For this review, use the dimensioned drawing (mm, ordinates from the lowest corner) and the shaded views. A direction names the side the tool comes from. Give positions to 0.01 mm unless a question says otherwise; leave off trailing zeros. Loops run counter-clockwise (first coordinate to the right, second up) from the corner with the lowest first, then second, coordinate; pieces in that order, holes last. Notation, with made-up numbers: (67.5, 84.25) - (94.5, 84.25) arc R19 ccw to (94.5, 115.25) - close; hole circle Ø3 at (-36, 7). An arc over 180 degrees is marked (long way). Put each result on its own line as item: value.
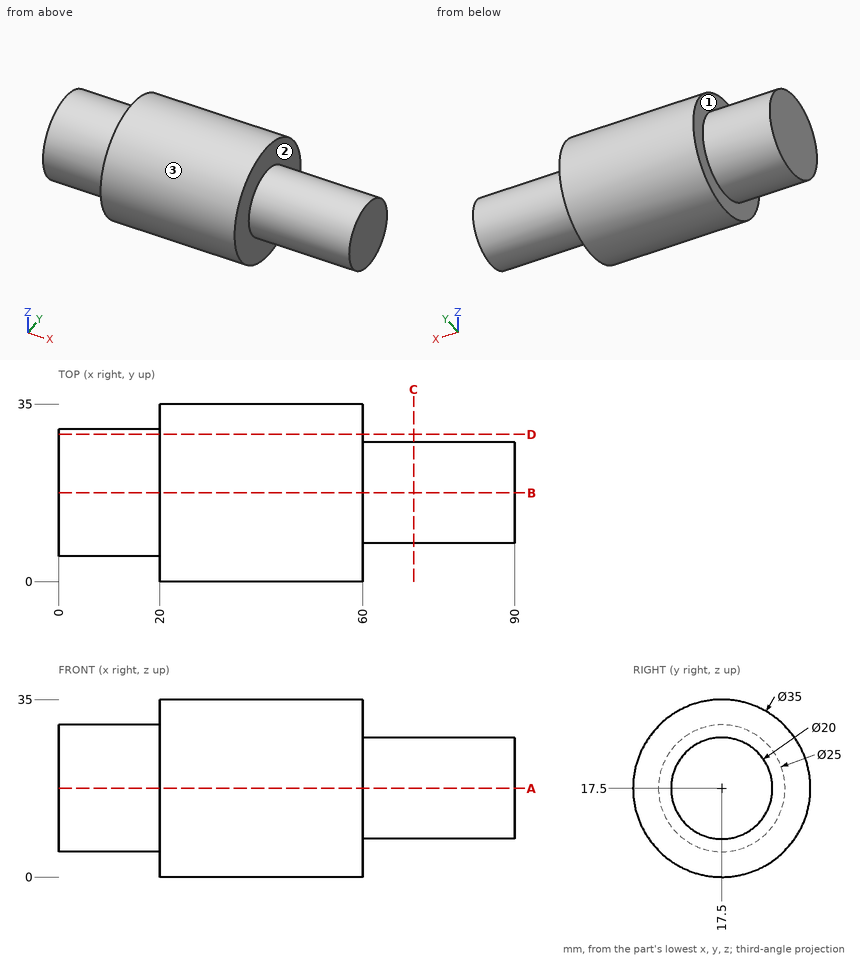
1) For the marked faces 1, 2 and 3, list the 3-axis set-ups (+Z, -Z, +X, -X, +Y, -Y) from which the entire face can be reached by the end or side of a thin tool; tool diameter is ignored.
Geometry check:
face 1: -X
face 2: +X
face 3: +X, -X
2) Take a section at A-A on z = 17.5. State the section outline as (x, y) points, and give its area (3 significant figures).
Geometry check:
outline: (0, 5) - (20, 5) - (20, 0) - (60, 0) - (60, 7.5) - (90, 7.5) - (90, 27.5) - (60, 27.5) - (60, 35) - (20, 35) - (20, 30) - (0, 30) - close
area: 2,500 mm²
3) Take a section at D-D on y = 29. State the section outline as (x, z) points, and give its area (3 significant figures).
Geometry check:
outline: (0, 12.6) - (20, 12.6) - (20, 4.31) - (60, 4.31) - (60, 30.69) - (20, 30.69) - (20, 22.4) - (0, 22.4) - close
area: 1,250 mm²
4) Insertion check: pin 1 Ø4 at (y, z) = (14.5, 20) entering from -X; pin 2 Ø1 at (x, y) = (26, 27) entering from -Z; pin 3 Ø2 at (x, y) = (46.5, 14) entering from -Z; pin 4 Ø6 at (x, y) = (15.5, 16.5) entering from +Z. Each pin has a flat end and moves straight along its axis. Give the tip position at first contact, or say it passes through.
Geometry check:
pin 1: stops at x = 0
pin 2: stops at z = 2.49
pin 3: stops at z = 0.18
pin 4: stops at z = 30
5) Wall thickness on line 1 (Z direction, x = 45, y = 17.5); line 2 (X direction, y = 16.5, z = 32.5); line 3 (Z direction, x = 15, y = 17): over which ranges is each line inside the solid? List them lowest first.
Geometry check:
line 1: z = 0 to 35
line 2: x = 20 to 60
line 3: z = 5.01 to 29.99
6) Take a section at C-C on x = 70. State the section outline as (y, z) points, and give its area (3 significant figures).
Geometry check:
outline: circle Ø20 at (17.5, 17.5)
area: 314 mm²
